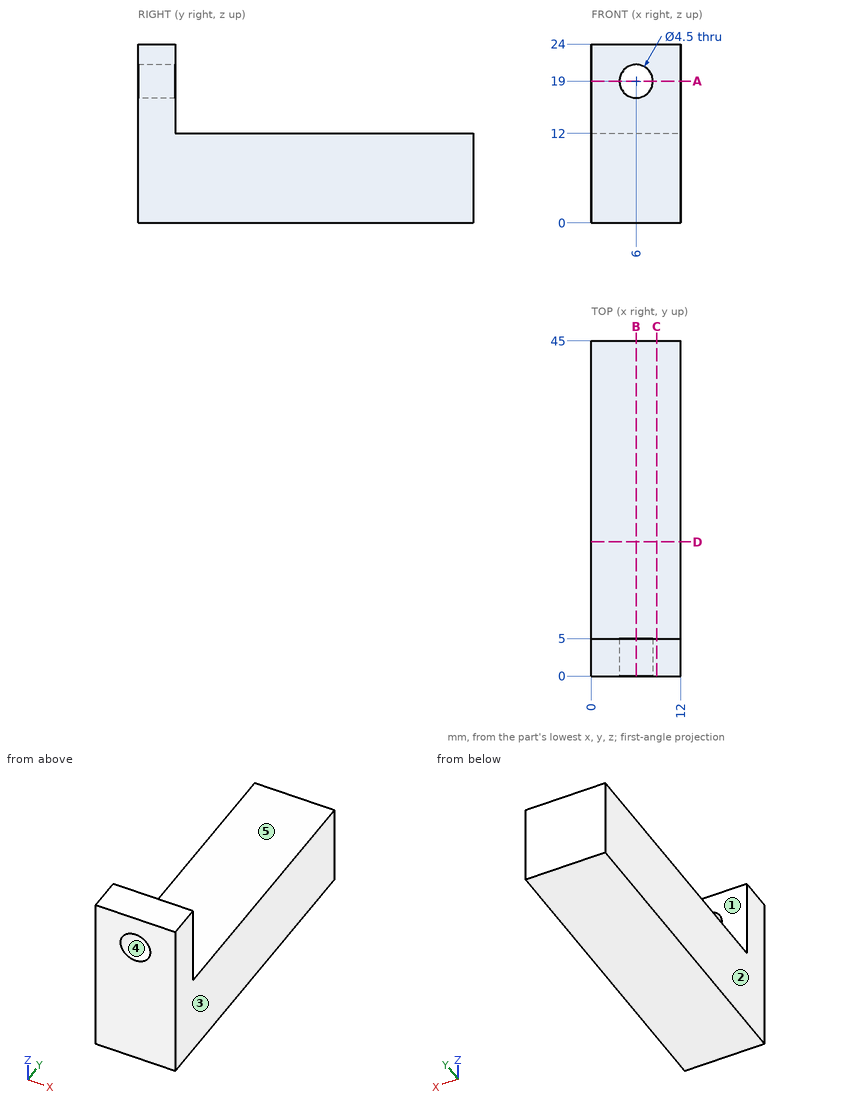
Design review of the part shown in the three views and the two pictorial views. Dimensions are in mm from the part's minimum x, y and z. A direction names the side the tool comes from. Round coordinates to 2 decimals unless told otherwise and drop trailing zeros. Write each loop counter-clockwise with the first axis right and the second up, starting at its lowest first coordinate (ties: lowest second). Pieces come first, ordered by that corner, then holes. Notation, with made-up numbers: (3, 30) -> (10, 30) arc R24 ccw to (10, 68) -> close; hole circle Ø3 at (-2, 24). An arc over 180 degrees is marked (long way). Answer as a JSON object with one key per item and string values.
1. Clearance check with flat-ended pins moving along their axes: pin 1 (12 mm diameter, centred on y = 39.5, z = 21, fed in from -X); pin 2 (6 mm diameter, centred on x = 4.5, z = 16.5, fed in from +Y); pin 3 (1.5 mm diameter, centred on x = 9.5, y = 38, fed in from +Z). State where each tip first meets the part, or that it passes through.
Results found:
{"pin 1": "passes through", "pin 2": "stops at y = 5", "pin 3": "stops at z = 12"}
2. The part is to be moulded in two halves that separate along X. For the marked faces 3, 4 and 5, say which applies: pulls with the +X half, pulls with the -X half, needs draft (parallel to the pull), parting line crosses it, or undercut.
Results found:
{"face 3": "pulls with the +X half", "face 4": "undercut", "face 5": "needs draft"}
3. To check wall thickness, follow line 1 along Z through (x, y) = (6, 3.85); line 2 along X through (y, z) = (2.2, 19); line 3 along Z through (x, y) = (7.75, 6). State the ranges of each line that lie inside material, in increasing order.
Results found:
{"line 1": "z = 0 to 16.75, 21.25 to 24", "line 2": "x = 0 to 3.75, 8.25 to 12", "line 3": "z = 0 to 12"}
4. Machinability: for the marked faces 1 and 2, which of the approach directions +Z, -Z, +X, -X, +Y, -Y give a long, thin tool a straight path to every point of the face, cutting with its end or side? Answer none if there is none.
Results found:
{"face 1": "+Z, +X, -X, +Y", "face 2": "+Z, -Z, -X, +Y, -Y"}
5. We need section A-A on z = 19. State the section outline as (x, y) points, and give its area (3 significant figures).
Results found:
{"outline": "(0, 0) -> (3.75, 0) -> (3.75, 5) -> (0, 5) -> close; (8.25, 0) -> (12, 0) -> (12, 5) -> (8.25, 5) -> close", "area": "37.5 mm^2"}
6. We need section D-D on y = 18. State the section outline as (x, z) points, and give its area (3 significant figures).
Results found:
{"outline": "(0, 0) -> (12, 0) -> (12, 12) -> (0, 12) -> close", "area": "144 mm^2"}
7. We need section C-C on x = 8.75. State the section outline as (y, z) points.
Results found:
{"outline": "(0, 0) -> (45, 0) -> (45, 12) -> (5, 12) -> (5, 24) -> (0, 24) -> close"}
8. We need section B-B on x = 6. State the section outline as (y, z) points.
Results found:
{"outline": "(0, 0) -> (45, 0) -> (45, 12) -> (5, 12) -> (5, 16.75) -> (0, 16.75) -> close; (0, 21.25) -> (5, 21.25) -> (5, 24) -> (0, 24) -> close"}
